Check sheet for the drawn part. Datum: minimum x, y, z corner. Units: mm. A direction names the side the tool comes from. Round coordinates to 2 decimals unless told otherwise and drop trailing zeros. Write each loop counter-clockwise with the first axis right and the second up, starting at its lowest first coordinate (ties: lowest second). Pieces come first, ordered by that corner, then holes. Notation, with made-up numbers: M 80.5,-38 L 104.5,-38 A32 cw 104.5,-10 Z; hole C -18,-1.75 d6. An arc over 180 degrees is marked long. Use a Markdown table: item, result.
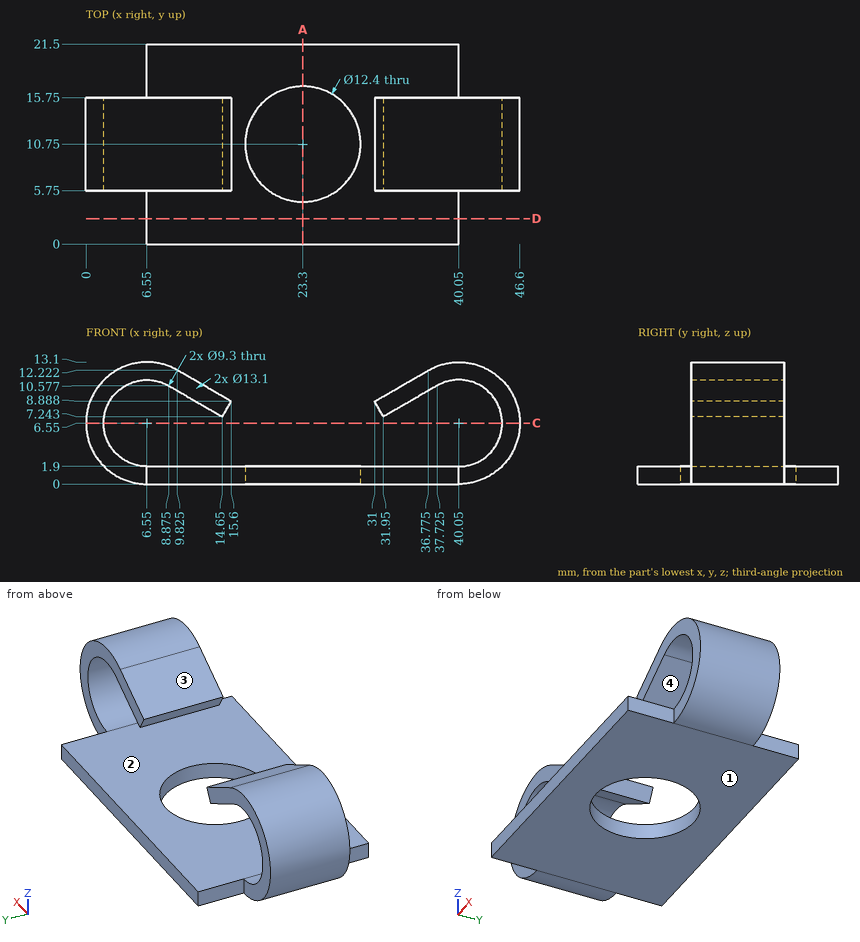
Item 1: Cross-section at A-A, the plane x = 23.3. Record the cut outline in (y, z), and give its area (3 significant figures).
Outcome:
| item | result |
|---|---|
| outline | M 0,0 L 4.55,0 L 4.55,1.9 L 0,1.9 Z; M 16.95,0 L 21.5,0 L 21.5,1.9 L 16.95,1.9 Z |
| area | 17.3 mm2 |
Item 2: Cross-section at C-C, the plane z = 6.55. Record the cut outline in (x, y), and give its area (3 significant figures).
Outcome:
| item | result |
|---|---|
| outline | M 0,5.75 L 1.9,5.75 L 1.9,15.75 L 0,15.75 Z; M 44.7,5.75 L 46.6,5.75 L 46.6,15.75 L 44.7,15.75 Z |
| area | 38.0 mm2 |
Item 3: Mould release check, pull along X, two halves, no side actions. Record for the marked faces 1 and 2: +X half, -X half, draft (parallel to the pull), parting line (faces both ways), or undercut.
Outcome:
| item | result |
|---|---|
| face 1 | draft |
| face 2 | undercut |
Item 4: Cross-section at D-D, the plane y = 2.75. Record the cut outline in (x, z).
Outcome:
| item | result |
|---|---|
| outline | M 6.55,0 L 40.05,0 L 40.05,1.9 L 6.55,1.9 Z |
Item 5: Access from +Z, -Z, +X, -X, +Y, -Y to the whole of each face (thin tool, end or side, straight path). Record for the marked faces 3 and 4.
Outcome:
| item | result |
|---|---|
| face 3 | +Z, +Y, -Y |
| face 4 | +Y, -Y |
Item 6: Material ranges on line 1 along Y through (x, z) = (23.3, 0.6); line 2 along Z through (x, y) = (40.05, 11.5); line 3 along X through (y, z) = (12.5, 6.55), recorded low to high. Write a range as from..to.
Outcome:
| item | result |
|---|---|
| line 1 | y = 0..4.55, 16.95..21.5 |
| line 2 | z = 0..1.9, 11.2..13.1 |
| line 3 | x = 0..1.9, 44.7..46.6 |
Item 7: Go/stop test with flat-tipped pins: pin 1 (5 mm diameter, centred on x = 5.5, z = 10, fed in from -Y); pin 2 (1.5 mm diameter, centred on y = 6, z = 9.5, fed in from +X); pin 3 (4 mm diameter, centred on x = 15.5, y = 5, fed in from +Z). Record where each tip stops, or that it passes through.
Outcome:
| item | result |
|---|---|
| pin 1 | stops at y = 5.75 |
| pin 2 | stops at x = 46.22 |
| pin 3 | stops at z = 10.02 |
